Read the model definition and answer for the solid it produces. Units are mm, in the model's axes. A direction names the side the tool comes from. Coordinates: 2 decimals unless noted, no trailing zeros. Order: outer loops, then holes, each group sorted by start corner. A loop starts at its lowest first (then second) coordinate and runs counter-clockwise, first axis right, second up. Notation, with made-up numbers: M 33,57 L 68,57 A23 ccw 68,94 Z; hole C -0.5,42 d1. An arc over 180 degrees is marked long. Put each result on its own line as item: value.
from build123d import *

# Parameters (mm, degrees)
F0_R          = 22.225
F1_DEPTH      = 40.64
F2_R          = 3.81
F3_DEPTH      = 40.641
F4_R          = 3.81
F5_DEPTH      = 22.226
F5_DEPTH_BACK = 22.226
F6_R          = 3.81
F7_DEPTH      = 22.2260001
F7_DEPTH_BACK = 22.2260001
F8_R          = 3.302
F9_DEPTH      = 40.6410001
F10_R         = 19.177
F11_DEPTH     = 38.735
F12_R         = 5.08


with BuildPart() as f1:
    # F0 (on Top) → F1 (new body)
    with BuildSketch(Plane.XY):
        Circle(F0_R)
    extrude(amount=-F1_DEPTH)

    # F2 (on face) → F3 (cut, through all)
    with BuildSketch(Plane(origin=(0, 0, -40.64), x_dir=(1, 0, 0), z_dir=(0, 0, -1))):
        Circle(F2_R)
    extrude(amount=-F3_DEPTH, mode=Mode.SUBTRACT)

    # F4 (on Right) → F5 (cut, two sides)
    with BuildSketch(Plane.YZ) as f5_sk:
        with Locations((0, -10.16)):
            Circle(F4_R)
    extrude(amount=-F5_DEPTH, mode=Mode.SUBTRACT)
    extrude(f5_sk.sketch, amount=F5_DEPTH_BACK, mode=Mode.SUBTRACT)

    # F6 (on Front) → F7 (cut, two sides)
    with BuildSketch(Plane.XZ) as f7_sk:
        with Locations((0, -10.16)):
            Circle(F6_R)
    extrude(amount=-F7_DEPTH, mode=Mode.SUBTRACT)
    extrude(f7_sk.sketch, amount=F7_DEPTH_BACK, mode=Mode.SUBTRACT)

    # F8 (on face) → F9 (cut, through all)
    with BuildSketch(Plane(origin=(0, 0, -40.64), x_dir=(1, 0, 0), z_dir=(0, 0, -1))):
        with Locations((10.922, 0)):
            Circle(F8_R)
        with Locations((-10.8710342307, 0)):
            Circle(F8_R)
    extrude(amount=-F9_DEPTH, mode=Mode.SUBTRACT)

    # F10 (on face) → F11 (cut)
    with BuildSketch(Plane.XY):
        Circle(F10_R)
    extrude(amount=-F11_DEPTH, mode=Mode.SUBTRACT)

    # F12
    f12_edges = [f1.edges().sort_by_distance(p)[0] for p in [
        (-22.225, 0, -40.64),
    ]]
    fillet(f12_edges, radius=F12_R)


solid = f1.part
Q1. Find section B-B on z = -10.16. Write down the section's boundary in (x, y) (3 decimals).
Answers below:
outline: M -21.896,-3.81 A22.225 ccw -3.81,-21.896 L -3.81,-18.795 A19.177 cw -18.795,-3.81 Z; M -21.896,3.81 L -18.795,3.81 A19.177 cw -3.81,18.795 L -3.81,21.896 A22.225 ccw Z; M 3.81,-21.896 A22.225 ccw 21.896,-3.81 L 18.795,-3.81 A19.177 cw 3.81,-18.795 Z; M 3.81,18.795 A19.177 cw 18.795,3.81 L 21.896,3.81 A22.225 ccw 3.81,21.896 Z
Q2. Find section A-A on y = 0. Give the number of separate pieces and of enclosed holes in the cut face, plus the area to 3 significant figures.
Answers below:
separate pieces: 6
enclosed holes: 0
area: 224 mm^2
Q3. Consider line 1 along Z through (x, y) = (-8.5, 3) (3 decimals); line 2 along X through (y, z) = (-5.5, -28); line 3 along Y through (x, z) = (17.5, -34). Determine where each line is inside the solid, lowest interval first.
Answers below:
line 1: z = -40.64 to -38.735
line 2: x = -21.53 to -18.37, 18.37 to 21.53
line 3: y = -13.7 to -7.84, 7.84 to 13.7
Q4. Given pin 1 (1 mm diameter, centred on x = -14, y = 14, fed in from -Z); pin 2 (1.5 mm diameter, centred on x = 3.5, z = -18, fed in from -Y); pin 3 (6 mm diameter, centred on x = 0, z = -10.16, fed in from +Y); pin 4 (6 mm diameter, centred on y = 10.5, z = -16, fed in from +X), each flat-ended and moving along its own axis, determine where each tip first touches the part or whether it passes through.
Answers below:
pin 1: stops at z = -40.16
pin 2: stops at y = -22.05
pin 3: passes through
pin 4: stops at x = 20.92
Q5. A tool of negligible diameter and unlimited length cuts with its end or side. For faces 5 (the face through (8.849, -17.013, -19.096)), 6 (the face through (8.3, 2.01, -39.7)), from which of +Z, -Z, +X, -X, +Y, -Y can it reach the whole face along a straight path? Write none if from no direction.
Answers below:
face 5: +Z
face 6: +Z, -Z
Q6. For a pull along Z with two mould halves and no side action, classify faces 1 (the face through (20.49, -3.02, -12.48)), 2 (the face through (0, 4, -40.64)), 3 (the face through (-14.17, -0.15, -39.7)), 4 (the face through (0, -4, -38.735)) as +Z half, -Z half, draft (parallel to the pull), parting line (faces both ways), or undercut.
Answers below:
face 1: undercut
face 2: -Z half
face 3: draft
face 4: +Z half
Q7. Find section C-C on z = -2.5. Write down the section's boundary in (x, y) (3 decimals), plus the area to 3 significant figures.
Answers below:
outline: C 0,0 d44.45; hole C 0,0 d38.354
area: 396 mm^2
